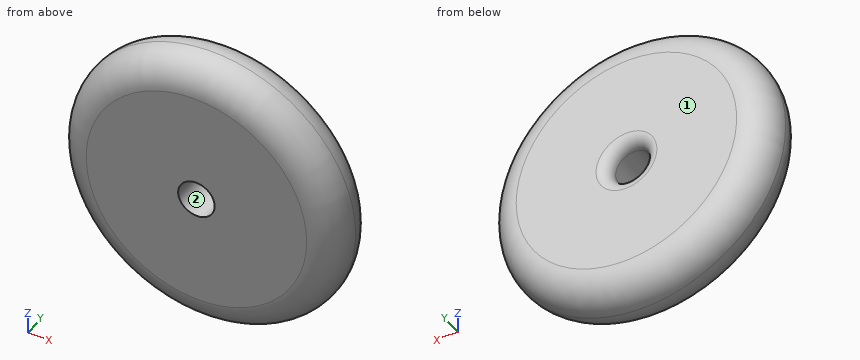
```python
from build123d import *

# Parameters (mm, degrees)
F0_R     = 23.125
F0_R_2   = 3
F1_DEPTH = 10
F2_R     = 4.99999
F3_R     = 2


# Not quite as in the source:
# - a fillet or chamfer is up to 0.001 mm smaller than in the source, because OpenCascade refuses the exact size


with BuildPart() as f1:
    # F0 (on Front) → F1 (new body)
    with BuildSketch(Plane.XZ):
        Circle(F0_R)
        Circle(F0_R_2, mode=Mode.SUBTRACT)
    extrude(amount=F1_DEPTH)

    # F2 (radius 5 in the source; OpenCascade refuses exactly that, so slightly less here)
    f2_edges = [f1.edges().sort_by_distance(p)[0] for p in [
        (-23.125, 0, 0),
        (-23.125, -10, 0),
    ]]
    fillet(f2_edges, radius=F2_R)

    # F3
    f3_edges = [f1.edges().sort_by_distance(p)[0] for p in [
        (-3, 0, 0),
        (-18.12501, 0, 0),
    ]]
    fillet(f3_edges, radius=F3_R)


solid = f1.part
```
Part model, mm, in its own coordinate system. Face numbers are marked on the shaded views. Round coordinates to 2 decimals unless told otherwise and drop trailing zeros. Loops run counter-clockwise (first coordinate to the right, second up) from the corner with the lowest first, then second, coordinate; pieces in that order, holes last. Notation, with made-up numbers: (-32, 60.25) -> (1, 60.25) arc R35 ccw to (1, 96.25) -> close; hole circle Ø1 at (16, 78). An arc over 180 degrees is marked (long way). Use a Markdown table: item, result.
1) Pull direction Z, two halves, no side cores. Call the marked faces 1 and 2: pulls with the +Z half, pulls with the -Z half, needs draft (parallel to the pull), parting line crosses it, or undercut.
The answers:
| item | result |
|---|---|
| face 1 | needs draft |
| face 2 | undercut |
2) Cut at D-D, the plane y = -1. List the corners of the cut face in (x, z) (3 decimals).
The answers:
| item | result |
|---|---|
| outline | circle Ø42.25 at (0, 0); hole circle Ø6.536 at (0, 0) |
3) Drop flat-ended pins along their axis: pin 1 Ø5 at (x, y) = (2.5, -2) entering from +Z; pin 2 Ø1.5 at (y, z) = (-5, -2.5) entering from -X; pin 3 Ø1 at (x, z) = (-12.5, -18.5) entering from +Y. Give the stop position or say it passes through.
The answers:
| item | result |
|---|---|
| pin 1 | stops at z = 23.03 |
| pin 2 | stops at x = -23.06 |
| pin 3 | stops at y = -1.64 |
4) Probe line 1 (Z direction, x = 0, y = -5.25); line 2 (Z direction, x = 2, y = -3.25); line 3 (X direction, y = -3.5, z = -14.5). List the from-to ranges inside material, lowest first. Write a range as [from, to].
The answers:
| item | result |
|---|---|
| line 1 | z = [-23.12, -3], [3, 23.12] |
| line 2 | z = [-22.72, -2.24], [2.24, 22.72] |
| line 3 | x = [-17.72, 17.72] |
5) Cut at C-C, the plane y = -4.25. List the corners of the cut face in (x, z), and give its area (3 significant figures).
The answers:
| item | result |
|---|---|
| outline | circle Ø46.14 at (0, 0); hole circle Ø6 at (0, 0) |
| area | 1,640 mm2 |
